Geometry: final body of the model. Coordinates: model frame, mm. A direction names the side the tool comes from. Round coordinates to 2 decimals unless told otherwise and drop trailing zeros. Write each loop counter-clockwise with the first axis right and the second up, starting at its lowest first coordinate (ties: lowest second). Pieces come first, ordered by that corner, then holes. Notation, with made-up numbers: M 63,40.5 L 122,40.5 A20 cw 122,57.5 Z; hole C -38.75,71.5 d3. An arc over 180 degrees is marked long. Use one line per item in the form item = value. Start each with the question number.
Item 1: Pin query (flat end, axial travel): pin 1 Ø2 at (y, z) = (11, 168.5) entering from +X; pin 2 Ø6 at (x, y) = (10, -24) entering from +Z (3 decimals). Return the tip coordinate at first contact, or that it passes through.
Item 2: Ray query, probe 1 along X at (y, z) = (11, 170); probe 2 along Y at (x, z) = (19, 107); probe 3 along Y at (x, z) = (17, 78). Return the intervals inside material, ascending.
Item 3: Reachability of faces 4 (the flat face through (3, 0, 0)), 5 (the cylindrical face through (6.07, 28.51, 141.95)) from +Z, -Z, +X, -X, +Y, -Y: full face, straight path, thin tool, end or side. Return the list, or none.
Item 4: Section query B-B (z = -7.5). Return loops of the section in (x, y), and give its area (3 significant figures).
Item 5: Section query A-A (x = 23). Return loops of the section in (y, z), and give its area (3 significant figures).
Item 6: Pull-direction query (Y, two-part tool) for faces 1 (the flat face through (4.07, 0, 146)), 2 (the flat face through (21, -40, 178)), 3 (the flat face through (3, 0, 320)); classes: pulls with the +Y half, pulls with the -Y half, needs draft (parallel to the pull), parting line crosses it, or undercut.
Item 7: Section query C-C (y = -6). Return loops of the section in (x, z).
Item 8: Section query D-D (x = 7.5). Return loops of the section in (y, z).
Autodesk Inventor part; units mm, degrees
ref_plane "Начальная плоскость" through (0, 0, -40) normal (0, 0, 1) x (1, 0, 0)
ref_plane "Конечная плоскость" through (0, 0, 320) normal (0, 0, 1) x (1, 0, 0)
ref_plane "РабПлоскость4" through (21.07, 40, -40) normal (0, -0.7071, -0.7071) x (1, 0, 0)
ref_plane "Начальная плоскость" through (0, 0, -40) normal (0, 0, 1) x (1, 0, 0)
ref_plane "Конечная плоскость" through (0, 0, 320) normal (0, 0, 1) x (1, 0, 0)
sketch "Эскиз" plane through (0, 0, 0) normal (0, 0, 1) x (1, 0, 0)
  line L0 (-1.43, 0) -> (-1.43, 40)
  line L1 (-1.43, 40) -> (43.57, 40)
  line L2 (43.57, 40) -> (43.57, 38.1774)
  line L3 (39.9881, 34.1993) -> (11.2338, 31.1771)
  line L4 (4.07, 23.221) -> (4.07, 0)
  line L5 (4.07, 0) -> (-1.43, 0) construction
  line L6 (23.82, 40) -> (23.82, 32.5) construction
  line L7 (43.57, 34.5758) -> (43.57, 32.5) construction
  line L8 (43.57, 32.5) -> (23.82, 32.5) construction
  line L9 (0, 15) -> (0, -27) construction
  line L10 (-5.539, 0) -> (16.0067, 0) construction
  line L11 (-1.43, 0) -> (-1.43, -40)
  line L12 (-1.43, -40) -> (43.57, -40)
  line L13 (43.57, -40) -> (43.57, -38.1774)
  line L14 (39.9881, -34.1993) -> (11.2338, -31.1771)
  line L15 (4.07, -23.221) -> (4.07, 0)
  arc A0 (11.2338, 31.1771) -> (4.07, 23.221) centre (12.07, 23.221) ccw
  arc A1 (4.07, -23.221) -> (11.2338, -31.1771) centre (12.07, -23.221) ccw
  arc A2 (39.9881, 34.1993) -> (43.57, 38.1774) centre (39.57, 38.1774) ccw
  arc A3 (43.57, -38.1774) -> (39.9881, -34.1993) centre (39.57, -38.1774) ccw
  line L16 (0, 56) -> (0, -56) construction
  line L17 (-15.5135, 0) -> (54.308, 0) construction
  point P0 (4.07, 30.4242)
  point P1 (43.57, -34.5758)
  point P2 (4.07, -30.4242)
  point P3 (23.82, -40)
  point P4 (23.82, -32.5)
  dimension "d0" = 5.5
  dimension "d1" = 40
  dimension "d2" = 45
  dimension "d3" = 7.5
  dimension "d4" = 19.75
  dimension "d5" = 2.0758
  dimension "d23" = 8
  dimension "d24" = 4
  dimension "d25" = 1.43
extrude "Тело" add sketch "Эскиз" along normal up to surface (360 mm away) from surface at -40
sketch "Sketch3" plane through (0, 0, 0) normal (0, 0, 1) x (1, 0, 0)
  line L0 (0, 0) -> (10, 0)
ref_plane "Work Plane3" through (0, 0, 0) normal (0, -1, 0) x (1, 0, 0)
sketch "Sketch4" plane through (0, 0, 0) normal (0, -1, 0) x (1, 0, 0)
  line L0 (-2, -40) -> (12, -40)
  line L1 (-2, 320) -> (12, 320)
  dimension "d29" = 360
ref_plane "РабПлоскость4" through (21.07, 40, -40) normal (0, -0.7071, -0.7071) x (1, 0, 0)
split "Разделение1" plane through (21.07, 40, -40) removes the side toward (0, -0.7071, -0.7071)
equation "\"d0\" = G_T"
equation "\"d1\" = 0.5 * G_H"
equation "\"d2\" = G_W"
equation "\"d3\" = G_T1"
equation "\"d4\" = G_C"
equation "\"d23\" = G_IR"
equation "\"d24\" = G_ER"
equation "\"d25\" = ex"
equation "\"d6\" = G_L"
equation "\"G_W\" = 45"
equation "\"G_T\" = 5.5"
equation "\"G_T1\" = 7.5"
equation "\"G_NG\" = 0.105104"
equation "\"G_ER\" = 4"
equation "\"G_IR\" = 8"
equation "\"G_C\" = 19.75"
equation "\"G_L\" = d29"
equation "\"ex\" = 1.43"
equation "\"G_OFFSET_END\" = 0"
properties part number "ISO 657/11 - CH 80 x 8 - 360" material "Сталь, мягкая"
Working result:
q1.pin_1 = 4.07
q1.pin_2 = through
q2.probe_1 = -1.43 to 4.07
q2.probe_2 = -40 to -31.99, 31.99 to 40
q2.probe_3 = -40 to -31.78, 31.78 to 40
q3.face_4 = -Z, +X, -X, -Y
q3.face_5 = +Z, -Z, +X
q4.outline = M -1.43,7.5 L 4.07,7.5 L 4.07,23.22 A8 cw 11.23,31.18 L 39.99,34.2 A4 ccw 43.57,38.18 L 43.57,40 L -1.43,40 Z
q4.area = 483 mm²
q5.outline = M -40,40 L -32.41,32.41 L -32.41,320 L -40,320 Z; M 32.41,-32.41 L 40,-40 L 40,320 L 32.41,320 Z
q5.area = 4,860 mm²
q6.face_1 = undercut
q6.face_2 = pulls with the -Y half
q6.face_3 = needs draft
q7.outline = M -1.43,6 L 4.07,6 L 4.07,320 L -1.43,320 Z
q8.outline = M -40,40 L -29.79,29.79 L -29.79,320 L -40,320 Z; M 29.79,-29.79 L 40,-40 L 40,320 L 29.79,320 Z
